Autodesk Inventor part; units mm, degrees
ref_plane "YZ Plane" through (0, 0, 0) normal (1, 0, 0) x (0, 1, 0)
ref_plane "XZ Plane" through (0, 0, 0) normal (0, 1, 0) x (-1, 0, 0)
ref_plane "XY Plane" through (0, 0, 0) normal (0, 0, 1) x (1, 0, 0)
sketch "Sketch1" plane through (0, 0, 0) normal (0, 0, 1) x (1, 0, 0)
  line L0 (80, 13.1) -> (-80, 13.1)
  line L1 (-80, 13.1) -> (-80, -13.1)
  line L2 (-80, -13.1) -> (80, -13.1)
  line L3 (80, -13.1) -> (80, 13.1)
  line L4 (80, 13.1) -> (-80, -13.1) construction
  line L5 (-80, 13.1) -> (80, -13.1) construction
  point P0 (0, 0)
  dimension "d0" = 160
  dimension "d1" = 26.2
extrude "Extrusion1" add sketch "Sketch1" along normal blind 11
sketch "Sketch2" plane through (80, -13.1, 0) normal (1, 0, 0) x (0, 0, -1)
  line L0 (0, 0) -> (0, 26.2)
  line L1 (0, 26.2) -> (-11, 26.2)
  line L2 (-11, 0) -> (-11, 26.2)
  line L3 (0, 0) -> (-11, 0)
  line L4 (-11, 26.2) -> (-11, 0)
  line L5 (-11, 26.2) -> (-5, 26.2)
  line L6 (-5, 26.2) -> (-5, 23.2)
  line L7 (-5, 23.2) -> (-11, 23.2)
  line L8 (-11, 23.2) -> (-11, 26.2)
  line L9 (-11, 23.2) -> (-8, 23.2)
  line L10 (-8, 23.2) -> (-8, 20.2)
  line L11 (-8, 20.2) -> (-11, 20.2)
  line L12 (-11, 20.2) -> (-11, 23.2)
  line L13 (-11, 26.2) -> (-5, 26.2)
  line L14 (-5, 26.2) -> (-5, 10.2)
  line L15 (-5, 10.2) -> (-11, 10.2)
  line L16 (-11, 10.2) -> (-11, 26.2)
  line L17 (-11, 10.2) -> (-5, 10.2)
  line L18 (-5, 10.2) -> (-5, 13.2)
  line L19 (-5, 13.2) -> (-11, 13.2)
  line L20 (-11, 13.2) -> (-11, 10.2)
  line L21 (-11, 13.2) -> (-8, 13.2)
  line L22 (-8, 13.2) -> (-8, 16.2)
  line L23 (-8, 16.2) -> (-11, 16.2)
  line L24 (-11, 16.2) -> (-11, 13.2)
  point P0 (0, 13.1)
  point P1 (-11, 20.2)
  dimension "d4" = 6
  dimension "d5" = 3
  dimension "d6" = 3
  dimension "d7" = 3
  dimension "d8" = 16
  dimension "d9" = 3
  dimension "d10" = 3
  dimension "d11" = 3
extrude "Extrusion2" cut sketch "Sketch2" against normal blind 157 contours L14 L19 L22 L23 L2 L11 L10 L7
fillet "Fillet1" radius 2 5 edges at (80, 10.1, 11) (80, -5, 11) (-80, 0, 11) (80, 0, 0) (-80, 0, 0)
sketch "Sketch4" plane through (-78, -13.1, 0) normal (0, -1, 0) x (1, 0, 0)
  arc A0 (-2, 2) -> (0, 0) centre (0, 2) ccw
  line L0 (0, 0) -> (156, 0)
  arc A1 (156, 0) -> (158, 2) centre (156, 2) ccw
  line L1 (158, 2) -> (158, 9)
  arc A2 (158, 9) -> (156, 11) centre (156, 9) ccw
  line L2 (0, 11) -> (156, 11)
  arc A3 (0, 11) -> (-2, 9) centre (0, 9) ccw
  line L3 (-2, 2) -> (-2, 9)
  circle A4 centre (148, 5.5) radius 4.1
  circle A5 centre (141, 5.5) radius 2.15
  line L4 (141, 7.65) -> (144.5089, 7.65)
  line L5 (141, 3.35) -> (144.5089, 3.35)
  circle A6 centre (15, 5.5) radius 4.1
  circle A7 centre (8, 5.5) radius 2.15
  line L6 (8, 3.35) -> (11.5089, 3.35)
  line L7 (8, 7.65) -> (11.5089, 7.65)
  point P0 (78, 0)
  point P1 (158, 5.5)
  point P2 (12.2407, 8.5325)
  point P3 (8.4381, 3.3951)
  point P4 (11.1965, 3.9692)
  point P5 (-2, 5.5)
  dimension "d19" = 8.2
  dimension "d20" = 4.3
  dimension "d21" = 7
  dimension "d22" = 0
  dimension "d23" = 10
  dimension "d24" = 8.2
  dimension "d25" = 4.3
  dimension "d26" = 7
  dimension "d27" = 10
  dimension "d28" = 0
  dimension "d40" = 0
extrude "Extrusion4" cut sketch "Sketch4" against normal blind 5.2 contours A4 | A4 L5 A5 L4 | A5 | A6 | A6 L6 A7 L7 | A7
sketch "Sketch5" plane through (-78, -13.1, 0) normal (0, -1, 0) x (1, 0, 0)
  arc A0 (8, 7.65) -> (8, 3.35) centre (8, 5.5) ccw
  arc A1 (11.5089, 3.35) -> (11.5089, 7.65) centre (15, 5.5) ccw
  arc A2 (141, 7.65) -> (141, 3.35) centre (141, 5.5) ccw
  line L0 (141, 7.65) -> (144.5089, 7.65)
  arc A3 (144.5089, 3.35) -> (144.5089, 7.65) centre (148, 5.5) ccw
  line L1 (144.5089, 3.35) -> (141, 3.35)
  arc A4 (-2, 2) -> (0, 0) centre (0, 2) ccw
  line L2 (0, 0) -> (156, 0)
  arc A5 (156, 0) -> (158, 2) centre (156, 2) ccw
  line L3 (158, 2) -> (158, 9)
  arc A6 (158, 9) -> (156, 11) centre (156, 9) ccw
  line L4 (0, 11) -> (156, 11)
  arc A7 (0, 11) -> (-2, 9) centre (0, 9) ccw
  line L5 (-2, 2) -> (-2, 9)
  circle A8 centre (8, 5.5) radius 4.1
  line L6 (8, 9.6) -> (15, 9.6)
  line L7 (8, 1.4) -> (15, 1.4)
  arc A9 (11.5089, 3.35) -> (11.5089, 7.65) centre (15, 5.5) ccw
  circle A10 centre (141, 5.5) radius 4.1
  line L8 (141, 9.6) -> (148, 9.6)
  line L9 (148, 1.4) -> (141, 1.4)
  line L10 (8, 7.65) -> (11.5089, 7.65)
  line L11 (11.5089, 3.35) -> (8, 3.35)
  arc A11 (8, 7.65) -> (8, 3.35) centre (8, 5.5) ccw
  point P0 (78, 0)
  point P1 (19.1, 5.5)
  point P2 (19.1, 5.5)
  point P3 (5.85, 5.5)
  point P4 (138.85, 5.5)
  point P5 (12.4867, 2.2607)
  point P6 (12.4867, 8.7393)
  point P7 (96.275, 2.2698)
  point P8 (96.275, 8.7302)
  point P9 (5.85, 5.5)
  point P10 (144.4911, 7.65)
  point P11 (144.4911, 3.35)
  point P12 (11.4911, 3.35)
  point P13 (11.4911, 7.65)
  dimension "d32" = 8.2
  dimension "d33" = 0
  dimension "d35" = 8.2
  dimension "d36" = 0
  dimension "d42" = 0
  dimension "d43" = 0
extrude "Extrusion5" cut sketch "Sketch5" along normal blind 3.2 from surface at -5.2 contours L10 A8 L11 A0 | A0 L11 A8 L10 | A8 L6 A1 L10 | L11 A1 L7 A8 | L0 A10 L1 A2 | A2 L1 A10 L0 | A10 L8 A3 L0 | L1 A3 L9 A10
properties part number "module-slot" material "PC/ABS Plastic"
CAD build for the part. Positions are in the model's coordinates, mm. A direction names the side the tool comes from. Round coordinates to 2 decimals unless told otherwise and drop trailing zeros. Loops run counter-clockwise (first coordinate to the right, second up) from the corner with the lowest first, then second, coordinate; pieces in that order, holes last. Notation, with made-up numbers: M 17,-6.5 L 56,-6.5 A32 ccw 56,26.5 Z; hole C 20,7 d1. An arc over 180 degrees is marked long. Use a Markdown table: item, result. Add a question column.
(1) Drill centre lines: line 1 (X direction, y = -8.75, z = 5.5); line 2 (Z direction, x = -56, y = 8.75); line 3 (Z direction, x = 70, y = -11.15). Where is each one in solid material? Low to high.
(2) Pull direction Y, two halves, no side cores. Call faces 4 (the face through (1, 13.1, 5)), 5 (the face through (80, -0.2, 5.5)), 6 (the face through (58.9, -9.5, 5.4)), 7 (the face through (3, 10.1, 6)): +Y half, -Y half, draft (parallel to the pull), parting line (faces both ways), or undercut.
(3) Cut at A-A (x = 38.5). Give the cut face in (y, z), and give its area (3 significant figures).
(4) Which spindle directions (+Z, -Z, +X, -X, +Y, -Y) get a long thin tool onto all of the face, cutting with end or side? Do faces 1 (the face through (-58.9, -11.1, 5.4)), 2 (the face through (60.7, -11.1, 5.6)), 3 (the face through (3, 7.1, 9)). Say none if no direction does.
(5) Flat gauge pins, fed straight in: pin 1 (6.5 mm diameter, centred on x = -63, z = 5.5, fed in from -Y); pin 2 (3 mm diameter, centred on x = 0, y = 5, fed in from +Z); pin 3 (1 mm diameter, centred on y = 5.5, z = 8.5, fed in from +X). Where does each tip first touch, or does it go through?
Geometry says:
| question | item | result |
|---|---|---|
| 1 | line 1 | x = -80 to -74.1, -58.9 to 58.9, 74.1 to 80 |
| 1 | line 2 | z = 0 to 5, 8 to 11 |
| 1 | line 3 | z = 0 to 1.4, 9.6 to 11 |
| 2 | face 4 | +Y half |
| 2 | face 5 | draft |
| 2 | face 6 | undercut |
| 2 | face 7 | undercut |
| 3 | outline | M -13.1,0 L 13.1,0 L 13.1,11 L 7.1,11 L 7.1,8 L 10.1,8 L 10.1,5 L 0.1,5 L 0.1,8 L 3.1,8 L 3.1,11 L -13.1,11 Z |
| 3 | area | 246 mm² |
| 4 | face 1 | -Y |
| 4 | face 2 | none |
| 4 | face 3 | +Z, +X |
| 5 | pin 1 | stops at y = -7.9 |
| 5 | pin 2 | stops at z = 5 |
| 5 | pin 3 | stops at x = -77 |
